```python
from build123d import *

# Parameters (mm, degrees)
F0_R     = 25.4
F0_R_2   = 22.225
F1_DEPTH = 84.1502
F2_R     = 38.1
F3_DEPTH = 3.175
F4_R     = 36.5125
F5_DEPTH = 25.4
F7_R     = 3.175
F8_DEPTH = 12.7


with BuildPart() as f1:
    # F0 (on Front) → F1 (new body)
    with BuildSketch(Plane.XZ):
        Circle(F0_R)
        Circle(F0_R_2, mode=Mode.SUBTRACT)
    extrude(amount=F1_DEPTH)

    # F2 (on Front) → F3 (join)
    with BuildSketch(Plane.XZ):
        Circle(F2_R)
    extrude(amount=F3_DEPTH)

    # F4 (on face) → F5 (join)
    with BuildSketch(Plane(origin=(0, 0, 0), x_dir=(-1, 0, 0), z_dir=(0, 1, 0))):
        Circle(F4_R)
    extrude(amount=F5_DEPTH)

    # F7 (on offset) → F8 (join)
    with BuildSketch(Plane.XY.offset(19.05)):
        with Locations((0, -15.875)):
            Circle(F7_R)
        with Locations((0, -28.575)):
            Circle(F7_R)
        with Locations((0, -41.275)):
            Circle(F7_R)
        with Locations((0, -53.975)):
            Circle(F7_R)
        with Locations((0, -66.675)):
            Circle(F7_R)
        with Locations((0, -79.375)):
            Circle(F7_R)
    extrude(amount=F8_DEPTH)


solid = f1.part
```
Geometry check sheet. Reference: the model listing, model coordinates, mm. A direction names the side the tool comes from. Coordinates: 2 decimals unless noted, no trailing zeros. Write each loop counter-clockwise with the first axis right and the second up, starting at its lowest first coordinate (ties: lowest second). Pieces come first, ordered by that corner, then holes. Notation, with made-up numbers: M -36.5,-34 L -27.5,-34 A23 cw -27.5,-20 Z; hole C 17,88 d9. An arc over 180 degrees is marked long. One line per item, written item: value. Start each with the question number.
(1) Sectioned sample at B-B, the plane x = -27. Enter the section's corners in (y, z) (3 decimals), and give its area (3 significant figures).
(2) Release check for a two-part mould opening along X. For faces 5 (the face through (-34.826, 12.522, 10.967)), 6 (the face through (0, -54, 31.75)), 7 (the face through (-4.8, -43.1, -21.7)) record: released by +X, released by -X, zero draft, split by the parting line, or undercut.
(3) Sectioned sample at A-A, the plane z = 0. Enter the section's corners in (x, y) (1 decimal).
(4) Sectioned sample at D-D, the plane x = -17.5. Enter the section's corners in (y, z) (1 decimal).
(5) Tool access check on faces 1 (the face through (0, -16, 19.05)), 2 (the face through (-0.688, -31.674, 20.617)), 3 (the face through (-0.688, -44.374, 28.429)), 4 (the face through (0, -79, 31.75)). Record the directions out of +Z, -Z, +X, -X, +Y, -Y that give a thin tool (end or side, any length) a straight path to the whole face; none if there is none.
(6) Sectioned sample at C-C, the plane y = -4.5. Enter the section's corners in (x, z) (3 decimals), and give its area (3 significant figures).
(7) Depth check by flat-ended pin: pin 1 (5 mm diameter, centred on x = -0.5, y = -68, fed in from +Z); pin 2 (3 mm diameter, centred on x = -0.5, y = -41.5, fed in from -Z); pin 3 (5 mm diameter, centred on x = 10.5, y = -69, fed in from +Z). Enter the tip coordinate at first touch or a pass-through.
(8) Scan lines: line 1 along Z through (x, y) = (0, -19) (3 decimals); line 2 along Z through (x, y) = (0, -50.5) (3 decimals). Record each from-to range of solid material in increasing order. Write a range as [from, to].
Filled sheet:
1. outline: M -3.175,-26.881 L 0,-26.881 L 0,-24.58 L 25.4,-24.58 L 25.4,24.58 L 0,24.58 L 0,26.881 L -3.175,26.881 Z
1. area: 1,420 mm²
2. face 5: split by the parting line
2. face 6: zero draft
2. face 7: undercut
3. outline: M -38.1,-3.2 L -25.4,-3.2 L -25.4,-84.2 L -22.2,-84.2 L -22.2,-3.2 L 22.2,-3.2 L 22.2,-84.2 L 25.4,-84.2 L 25.4,-3.2 L 38.1,-3.2 L 38.1,0 L 36.5,0 L 36.5,25.4 L -36.5,25.4 L -36.5,0 L -38.1,0 Z
4. outline: M -84.2,-18.4 L -3.2,-18.4 L -3.2,-33.8 L 0,-33.8 L 0,-32 L 25.4,-32 L 25.4,32 L 0,32 L 0,33.8 L -3.2,33.8 L -3.2,18.4 L -84.2,18.4 L -84.2,13.7 L -3.2,13.7 L -3.2,-13.7 L -84.2,-13.7 Z
5. face 1: -Y
5. face 2: none
5. face 3: +Z
5. face 4: +Z, +X, -X, -Y
6. outline: C 0,0 d50.8; hole C 0,0 d44.45
6. area: 475 mm²
7. pin 1: z = 31.75
7. pin 2: z = -25.4
7. pin 3: z = 24.11
8. line 1: [-25.4, -22.225], [19.05, 31.75]
8. line 2: [-25.4, -22.225], [22.225, 25.4]
